from build123d import *

# Parameters (mm, degrees)
SKETCH1_R           = 25.4
SKETCH1_R_2         = 19.05
BOSS_EXTRUDE1_DEPTH = 50.8
SKETCH2_R           = 38.1
BOSS_EXTRUDE2_DEPTH = 76.2


with BuildPart() as part:
    # Sketch1 → Boss-Extrude1 (new body)
    # profile 1 of 2: a face of its own
    with BuildSketch(Plane(origin=(0, 0, 0), x_dir=(1, 0, 0), z_dir=(0, 1, 0))):
        with BuildLine():
            ThreePointArc((25.4, 0), (17.960512242, -17.960512242), (0, -25.4))
            Line((0, -25.4), (57.15, -25.4))
            Line((57.15, -25.4), (57.15, 25.4))
            Line((57.15, 25.4), (0, 25.4))
            ThreePointArc((0, 25.4), (17.960512242, 17.960512242), (25.4, 0))
        make_face()
    # profile 2 of 2: a face of its own
    with BuildSketch(Plane(origin=(0, 0, 0), x_dir=(1, 0, 0), z_dir=(0, 1, 0))):
        Circle(SKETCH1_R)
        with Locations(Location((0, 0, 0), (0, 0, 270))):
            Circle(SKETCH1_R_2, mode=Mode.SUBTRACT)
    extrude(amount=BOSS_EXTRUDE1_DEPTH)

    # Sketch2 → Boss-Extrude2 (add)
    with BuildSketch(Plane(origin=(57.15, 0, 0), x_dir=(0, 0, -1), z_dir=(1, 0, 0))):
        with Locations(Location((0, 25.4, 0), (0, 0, 180))):
            Circle(SKETCH2_R)
    extrude(amount=BOSS_EXTRUDE2_DEPTH)


solid = part.part
The listing builds one solid part. Answer for the finished solid, in the listing's coordinates (mm). A direction names the side the tool comes from. Coordinates: 2 decimals unless noted, no trailing zeros. Write each loop counter-clockwise with the first axis right and the second up, starting at its lowest first coordinate (ties: lowest second). Pieces come first, ordered by that corner, then holes. Notation, with made-up numbers: M 29.5,66.5 L 76.5,66.5 A22 cw 76.5,97.5 Z; hole C 0.25,11 d5. An arc over 180 degrees is marked long. Put each result on its own line as item: value. Start each with the question number.
1. A cutting plane is placed at B-B on y = 25.4. Write down the section's boundary in (x, z).
2. Flat-ended cylindrical pins translate along their axes: P1, Ø23, axis at y = 17, z = 2, coming from the -X side; P2, Ø3, axis at x = 9, y = 5, coming from the -Z side; P3, Ø3, axis at x = 79, z = 24, coming from the +Y side. Find the tip coordinate at first contact, or state that the pin passes through.
3. For a pull along X with two mould halves and no side action, classify faces 1 (the flat face through (24, 0, 0)), 2 (the flat face through (133.35, 25, -1)), 3 (the cylindrical face through (-11.59, 25.04, -15.12)), 4 (the cylindrical face through (-25.394, 25.044, -0.559)) as pulls with the +X half, pulls with the -X half, needs draft (parallel to the pull), parting line crosses it, or undercut.
4. A cutting plane is placed at D-D on x = 67.5. Write down the section's boundary in (y, z), then the cut area to 3 significant figures.
5. Which of the six approach directions +Z, -Z, +X, -X, +Y, -Y give full straight-line access (tool end or side, diameter ignored) to faces 5 (the flat face through (29, 25, -25.4)), 6 (the cylindrical face through (94.717, 62.594, -8.259)), 7 (the flat face through (28, 25, 25.4)), 8 (the flat face through (24, 50.8, 0))?
6. A cutting plane is placed at C-C on z = -22. Write down the section's boundary in (x, y).
7. Consider line 1 (X direction, y = 19.5, z = 0); line 2 (X direction, y = 23, z = 27.5); line 3 (Y direction, x = 43.5, z = 15.5). Determine where each line is inside the solid, lowest interval first. Write a range as from..to.
8. A cutting plane is placed at A-A on z = 0. Write down the section's boundary in (x, y).
Resolved:
1. outline: M 0,-25.4 L 57.15,-25.4 L 57.15,-38.1 L 133.35,-38.1 L 133.35,38.1 L 57.15,38.1 L 57.15,25.4 L 0,25.4 A25.4 ccw Z; hole C 0,0 d38.1
2. P1: stops at x = -25.4
2. P2: stops at z = -25.4
2. P3: stops at y = 56.15
3. face 1: needs draft
3. face 2: pulls with the +X half
3. face 3: undercut
3. face 4: pulls with the -X half
4. outline: C 25.4,0 d76.2
4. area: 4,560 mm2
5. face 5: -Z, -X, +Y, -Y
5. face 6: +X, -X
5. face 7: +Z, -X, +Y, -Y
5. face 8: +Z, -Z, -X, +Y
6. outline: M -12.69,0 L 57.15,0 L 57.15,-5.71 L 133.35,-5.71 L 133.35,56.51 L 57.15,56.51 L 57.15,50.8 L -12.69,50.8 Z
7. line 1: x = -25.4..-19.05, 19.05..133.35
7. line 2: x = 57.15..133.35
7. line 3: y = 0..50.8
8. outline: M -25.4,0 L -19.05,0 L -19.05,50.8 L -25.4,50.8 Z; M 19.05,0 L 57.15,0 L 57.15,-12.7 L 133.35,-12.7 L 133.35,63.5 L 57.15,63.5 L 57.15,50.8 L 19.05,50.8 Z
